```python
from build123d import *

# Parameters (mm, degrees)
SKETCH2_R            = 1.5
SKETCH2_W            = 25.4
SKETCH2_H            = 46
BOSS_EXTRUDE1_DEPTH  = 2
BOSS_EXTRUDE3_DEPTH  = 4.62
SKETCH5_5_R          = 1.5
CUT_EXTRUDE3_DEPTH   = 10
BOSS_EXTRUDE4_DEPTH  = 4.62
SKETCH8_W            = 140
SKETCH8_H            = 350
SKETCH8_W_2          = 35.6
SKETCH8_H_2          = 30
BOSS_EXTRUDE10_DEPTH = 4.63
SKETCH9_W            = 140
SKETCH9_H            = 350
SKETCH9_W_2          = 35.6
SKETCH9_H_2          = 30
BOSS_EXTRUDE11_DEPTH = 4.8
SKETCH10_R           = 2
CUT_EXTRUDE4_DEPTH   = 10.43


with BuildPart() as part:
    # Sketch2 → Boss-Extrude1 (new body)
    with BuildSketch(Plane(origin=(0, 0, 0), x_dir=(1, 0, 0), z_dir=(0, 1, 0))):
        Polygon((37.8, -65.8), (37.8, 64.2), (9.15, 64.2), (-37.8, 64.2), (-37.8, -65.8), align=None)
        with Locations((-8.5, -23.3)):
            Circle(SKETCH2_R, mode=Mode.SUBTRACT)
        with Locations((-15, -17)):
            Circle(SKETCH2_R, mode=Mode.SUBTRACT)
        with Locations((-15, 0)):
            Circle(SKETCH2_R, mode=Mode.SUBTRACT)
        with Locations((8.5, -23.3)):
            Circle(SKETCH2_R, mode=Mode.SUBTRACT)
        with Locations((15, -17)):
            Circle(SKETCH2_R, mode=Mode.SUBTRACT)
        with Locations((15, 0)):
            Circle(SKETCH2_R, mode=Mode.SUBTRACT)
        with Locations((-15, 17)):
            Circle(SKETCH2_R, mode=Mode.SUBTRACT)
        with Locations((0, 2)):
            Rectangle(SKETCH2_W, SKETCH2_H, mode=Mode.SUBTRACT)
        with Locations((15, 17)):
            Circle(SKETCH2_R, mode=Mode.SUBTRACT)
    extrude(amount=BOSS_EXTRUDE1_DEPTH)

    # Sketch5 → Boss-Extrude3 (add)
    with BuildSketch(Plane.XZ):
        Polygon((37.8, 30.8), (37.8, 65.8), (-37.8, 65.8), (-37.8, 30.8), (-37.8, -3), (-17.8, -3), (-17.8, 27), (17.8, 27), (17.8, -3), (37.8, -3), align=None)
    extrude(amount=BOSS_EXTRUDE3_DEPTH)

    # Sketch5<5> → Cut-Extrude3 (cut)
    with BuildSketch(Plane.XZ):
        Polygon((37.8, -3), (12.7, -3), (12.7, -25), (-12.7, -25), (-12.7, -3), (-37.8, -3), (-37.8, -64.2), (37.8, -64.2), align=None)
        with Locations((15, -17)):
            Circle(SKETCH5_5_R, mode=Mode.SUBTRACT)
        with Locations((-15, -17)):
            Circle(SKETCH5_5_R, mode=Mode.SUBTRACT)
    extrude(amount=-CUT_EXTRUDE3_DEPTH, mode=Mode.SUBTRACT)

    # Sketch6 → Boss-Extrude4 (add)
    with BuildSketch(Plane(origin=(0, 2, 0), x_dir=(1, 0, 0), z_dir=(0, 1, 0))):
        Polygon((-17.8, -25.996410493), (-17.8, 3), (-37.8, 3), (-37.8, -65.8), (0, -65.8), (37.8, -65.8), (37.8, 3), (17.8, 3), (17.8, -25.996410493), align=None)
    extrude(amount=BOSS_EXTRUDE4_DEPTH)

    # Sketch8 → Boss-Extrude10 (add)
    with BuildSketch(Plane.XZ.offset(4.62)):
        with Locations((0, -109.2)):
            Rectangle(SKETCH8_W, SKETCH8_H)
        with Locations((0, 12)):
            Rectangle(SKETCH8_W_2, SKETCH8_H_2, mode=Mode.SUBTRACT)
    extrude(amount=BOSS_EXTRUDE10_DEPTH)

    # Sketch9 → Boss-Extrude11 (add)
    with BuildSketch(Plane.XZ.offset(9.25)):
        with Locations((0, -109.2)):
            Rectangle(SKETCH9_W, SKETCH9_H)
        with Locations((0, 12)):
            Rectangle(SKETCH9_W_2, SKETCH9_H_2, mode=Mode.SUBTRACT)
    extrude(amount=BOSS_EXTRUDE11_DEPTH)

    # Sketch10 → Cut-Extrude4 (cut, through all)
    with BuildSketch(Plane(origin=(0, -4.62, 0), x_dir=(1, 0, 0), z_dir=(0, 1, 0))):
        with Locations((51.4, 57.95)):
            Circle(SKETCH10_R)
        with Locations((51.4, 159.2)):
            Circle(SKETCH10_R)
        with Locations((51.4, 259.2)):
            Circle(SKETCH10_R)
        with Locations((-51.4, 259.2)):
            Circle(SKETCH10_R)
        with Locations((-51.4, 57.95)):
            Circle(SKETCH10_R)
        with Locations((-51.4, 159.2)):
            Circle(SKETCH10_R)
    extrude(amount=-CUT_EXTRUDE4_DEPTH, mode=Mode.SUBTRACT)


solid = part.part
```
Input: part model. Units: mm. Frame: model coordinates. A direction names the side the tool comes from. Round coordinates to 2 decimals unless told otherwise and drop trailing zeros. Loops run counter-clockwise (first coordinate to the right, second up) from the corner with the lowest first, then second, coordinate; pieces in that order, holes last. Notation, with made-up numbers: (-26, 10) -> (25, 10) arc R12 ccw to (25, 20) -> close; hole circle Ø7 at (34.5, 14.25). An arc over 180 degrees is marked (long way). One line per item, written item: value.
(1) Section B-B (z = -118.5). Return the cut outline in (x, y), plus the area to 3 significant figures.
Geometry check:
outline: (-70, -14.05) -> (70, -14.05) -> (70, -4.62) -> (-70, -4.62) -> close
area: 1,320 mm2
(2) Mould query, pull axis Z, two halves, no side actions, for faces 1 (the face through (-70, -9, -112)), 2 (the face through (-17.8, -7, 12)), 3 (the face through (-1, -9, -284.2)). Classes: pulls with the +Z half, pulls with the -Z half, needs draft (parallel to the pull), parting line crosses it, or undercut.
Geometry check:
face 1: needs draft
face 2: undercut
face 3: pulls with the -Z half
(3) Set-up query: faces 4 (the face through (0, -9, -3)), 5 (the face through (0, 2, 22)), 6 (the face through (0, 0, 22)), 7 (the face through (-28, 1, -3)). Return all of +Z, -Z, +X, -X, +Y, -Y with unobstructed straight access to the full face (end or side cutting, diameter ignored); none if empty.
Geometry check:
face 4: -Y
face 5: -Z, +Y
face 6: -Z, -Y
face 7: -Z, +X, -X, +Y
(4) Material intervals for line 1 (Z direction, x = 51.4, y = -12); line 2 (X direction, y = 1.1, z = 23.3); line 3 (X direction, y = -11.25, z = -57.95), sorted ascending. Write a range as [from, to].
Geometry check:
line 1: [-284.2, -261.2], [-257.2, -161.2], [-157.2, -59.95], [-55.95, 65.8]
line 2: [-37.8, -10], [-7, 7], [10, 37.8]
line 3: [-70, -53.4], [-49.4, 49.4], [53.4, 70]
(5) Section A-A (y = -8.5). Return the cut outline in (x, z), plus the area to 3 significant figures.
Geometry check:
outline: (-70, -284.2) -> (70, -284.2) -> (70, 65.8) -> (-70, 65.8) -> close; hole circle Ø4 at (-51.4, -259.2); hole circle Ø4 at (-51.4, -159.2); hole circle Ø4 at (-51.4, -57.95); hole (-17.8, -3) -> (17.8, -3) -> (17.8, 27) -> (-17.8, 27) -> close; hole circle Ø4 at (51.4, -259.2); hole circle Ø4 at (51.4, -159.2); hole circle Ø4 at (51.4, -57.95)
area: 47,900 mm2
(6) Pin query (flat end, axial travel): pin 1 (8 mm diameter, centred on x = -36.5, z = -19, fed in from +Y); pin 2 (0.6 mm diameter, centred on y = 0.5, z = 6.5, fed in from -X); pin 3 (0.6 mm diameter, centred on y = 1.5, z = 7, fed in from +X). Return the tip coordinate at first contact, or that it passes through.
Geometry check:
pin 1: y = -4.62
pin 2: x = -37.8
pin 3: x = 37.8
